```python
from build123d import *

# Parameters (mm, degrees)
SKETCH2_W           = 48.26
SKETCH2_H           = 7.62
BOSS_EXTRUDE1_DEPTH = 2.54
SKETCH3_W           = 5.08
SKETCH3_H           = 10.16
BOSS_EXTRUDE2_DEPTH = 2.54
SKETCH4_R           = 1.016
CUT_EXTRUDE1_DEPTH  = 2.54
SKETCH5_W           = 7.62
SKETCH5_H           = 7.62
BOSS_EXTRUDE3_DEPTH = 2.54
SKETCH7_R           = 1.55
CUT_EXTRUDE2_DEPTH  = 2.54


with BuildPart() as part:
    # Sketch2 → Boss-Extrude1 (new body)
    with BuildSketch(Plane(origin=(0, 0, 0), x_dir=(1, 0, 0), z_dir=(0, 1, 0))):
        with Locations((24.13, 3.81)):
            Rectangle(SKETCH2_W, SKETCH2_H)
    extrude(amount=BOSS_EXTRUDE1_DEPTH)

    # Sketch3 → Boss-Extrude2 (add)
    with BuildSketch(Plane(origin=(0, 0, 0), x_dir=(1, 0, 0), z_dir=(0, 1, 0))):
        with Locations((-2.54, 5.08)):
            Rectangle(SKETCH3_W, SKETCH3_H)
    extrude(amount=BOSS_EXTRUDE2_DEPTH)

    # Sketch4 → Cut-Extrude1 (cut)
    with BuildSketch(Plane(origin=(0, 2.54, 0), x_dir=(1, 0, 0), z_dir=(0, 1, 0))):
        with Locations(Location((-2.608533825, 7.62, 0), (0, 0, 270))):
            Circle(SKETCH4_R)
    extrude(amount=-CUT_EXTRUDE1_DEPTH, mode=Mode.SUBTRACT)

    # Sketch5 → Boss-Extrude3 (add)
    with BuildSketch(Plane.ZY.offset(-48.26)):
        with Locations((-3.81, 6.35)):
            Rectangle(SKETCH5_W, SKETCH5_H)
    extrude(amount=BOSS_EXTRUDE3_DEPTH)

    # Sketch7 → Cut-Extrude2 (cut)
    with BuildSketch(Plane.ZY.offset(-45.72)):
        with Locations((-3.81, 6.35)):
            Circle(SKETCH7_R)
    extrude(amount=-CUT_EXTRUDE2_DEPTH, mode=Mode.SUBTRACT)


solid = part.part
```
Design review of the part built by this model. Coordinates are the model's own, in mm. A direction names the side the tool comes from. Coordinates: 2 decimals unless noted, no trailing zeros. Loops run counter-clockwise (first coordinate to the right, second up) from the corner with the lowest first, then second, coordinate; pieces in that order, holes last.
Q1. For pin 1 (4 mm diameter, centred on x = 33, y = 6, fed in from -Z); pin 2 (4 mm diameter, centred on y = 8, z = -6, fed in from -X); pin 3 (3 mm diameter, centred on x = 11, z = -6, fed in from +Y); pin 4 (0.8 mm diameter, centred on y = 1, z = -8.5, fed in from +X), all flat-tipped, find the tip position at first contact; note any pin that passes through.
Reported:
pin 1: passes through
pin 2: stops at x = 45.72
pin 3: stops at y = 2.54
pin 4: stops at x = 0
Q2. We need section D-D on x = 7.5. State the section outline as (y, z) points.
Reported:
outline: (0, -7.62) - (2.54, -7.62) - (2.54, 0) - (0, 0) - close
Q3. Tool access review of faces 1 (the face through (24, 2, 0)), 2 (the face through (0, 1, -9)), 3 (the face through (45.72, 6, -2)): name each direction out of +Z, -Z, +X, -X, +Y, -Y from which nothing blocks a thin tool from reaching the whole face with its end or side.
Reported:
face 1: +Z, +X, -X, +Y, -Y
face 2: -Z, +X, +Y, -Y
face 3: +Z, -Z, -X, +Y
Q4. The part is to be moulded in two halves that separate along Y. For faces 4 (the face through (26, 2, -7.62)), 5 (the face through (46.97, 5.41, -5.04)), 6 (the face through (47, 10.16, -4)), say which applies: +Y half, -Y half, draft (parallel to the pull), parting line (faces both ways), or undercut.
Reported:
face 4: draft
face 5: undercut
face 6: +Y half
Q5. We need section C-C on y = 2. State the section outline as (x, z) points.
Reported:
outline: (-5.08, -10.16) - (0, -10.16) - (0, -7.62) - (48.26, -7.62) - (48.26, 0) - (-5.08, 0) - close; hole circle Ø2.03 at (-2.61, -7.62)
Q6. We need section B-B on y = 6.35. State the section outline as (x, z) points, and give its area (3 significant figures).
Reported:
outline: (45.72, -7.62) - (48.26, -7.62) - (48.26, -5.36) - (45.72, -5.36) - close; (45.72, -2.26) - (48.26, -2.26) - (48.26, 0) - (45.72, 0) - close
area: 11.5 mm2
Q7. To check wall thickness, follow line 1 (Y direction, x = 46.55, z = -3.81); line 2 (Y direction, x = 18, z = -4.25); line 3 (X direction, y = 9.5, z = -4.75). State the ranges of each line that lie inside material, in increasing order.
Reported:
line 1: y = 0 to 4.8, 7.9 to 10.16
line 2: y = 0 to 2.54
line 3: x = 45.72 to 48.26
Q8. We need section A-A on z = -3.81. State the section outline as (x, y) points, and give its area (3 significant figures).
Reported:
outline: (-5.08, 0) - (48.26, 0) - (48.26, 4.8) - (45.72, 4.8) - (45.72, 2.54) - (-5.08, 2.54) - close; (45.72, 7.9) - (48.26, 7.9) - (48.26, 10.16) - (45.72, 10.16) - close
area: 147 mm2
